CAD build for the part. Positions are in the model's coordinates, mm. Give positions to 0.01 mm unless a question says otherwise; leave off trailing zeros. Loops run counter-clockwise (first coordinate to the right, second up) from the corner with the lowest first, then second, coordinate; pieces in that order, holes last. Notation, with made-up numbers: M 80.25,-3 L 97.25,-3 A28 ccw 97.25,33 Z; hole C 58.5,64.5 d1. An arc over 180 degrees is marked long. Answer as CSV lines item,"result".
```python
from build123d import *

# Parameters (mm, degrees)
SKETCH1_R          = 5.4864
BASE_EXTRUDE_DEPTH = 0.635
SKETCH2_R          = 4.064
CUT_EXTRUDE1_DEPTH = 1.635
CUT_EXTRUDE4_DEPTH = 1.635
CIRPATTERN1_COUNT  = 14


with BuildPart() as part:
    # Sketch1 → Base-Extrude (new body)
    with BuildSketch(Plane.XY):
        Circle(SKETCH1_R)
    extrude(amount=BASE_EXTRUDE_DEPTH)

    # Sketch2 → Cut-Extrude1 (cut, through all)
    with BuildSketch(Plane.XY.offset(0.635)):
        Circle(SKETCH2_R)
    extrude(amount=-CUT_EXTRUDE1_DEPTH, mode=Mode.SUBTRACT)

    # Sketch3 → Cut-Extrude4 (cut, through all)
    with BuildSketch(Plane.XY.offset(0.635)):
        with BuildLine():
            Line((0.381, 4.04610121), (0.381, 4.3815))
            ThreePointArc((0.381, 4.3815), (0, 4.7625), (-0.381, 4.3815))
            Line((-0.381, 4.3815), (-0.381, 4.04610121))
            ThreePointArc((-0.381, 4.04610121), (0, 4.064), (0.381, 4.04610121))
        make_face()
    cut_extrude4 = extrude(amount=-CUT_EXTRUDE4_DEPTH, mode=Mode.SUBTRACT)

    # CirPattern1: Cut-Extrude4 ×14 about axis
    cirpattern1_axis = Axis((0, 0, 0), (0, 0, 1))
    for i in range(1, CIRPATTERN1_COUNT):
        add(cut_extrude4.rotate(cirpattern1_axis, i * 360 / CIRPATTERN1_COUNT), mode=Mode.SUBTRACT)


solid = part.part
```
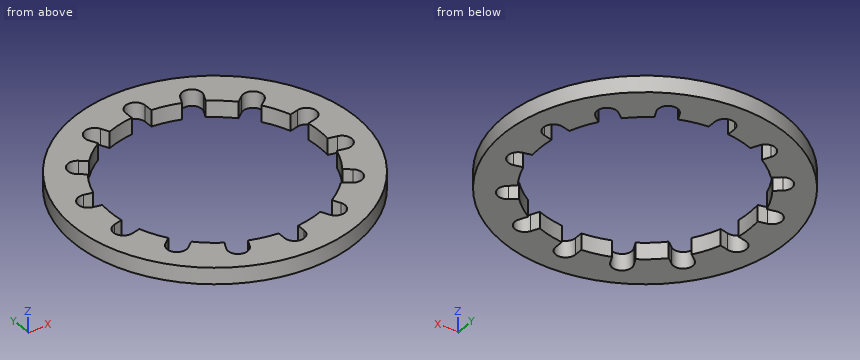
Q1. Wall check: line 1 (X direction, y = 4.25, z = 0.4); line 2 (X direction, y = 3.25, z = 0.2); line 3 (Y direction, x = -3.5, z = 0.45) (3 decimals). Give the ranges that are in metal, low to high. Write a range as [from, to].
Solution:
line 1,"x = [-3.47, -2.13], [-1.67, -0.38], [0.38, 1.67], [2.13, 3.47]"
line 2,"x = [-4.42, -2.44], [2.44, 4.42]"
line 3,"y = [-4.225, -3.105], [-2.304, -2.065], [2.065, 2.304], [3.105, 4.225]"
Q2. Cut at C-C (x = -4.5). Write the cut outline in (y, z) (3 decimals).
Solution:
outline,"M -3.139,0 L -1.28,0 L -1.28,0.635 L -3.139,0.635 Z; M -0.67,0 L 0.67,0 L 0.67,0.635 L -0.67,0.635 Z; M 1.28,0 L 3.139,0 L 3.139,0.635 L 1.28,0.635 Z"
Q3. Cut at B-B (y = 0). Write the cut outline in (x, z) (3 decimals).
Solution:
outline,"M -5.486,0 L -4.064,0 L -4.064,0.635 L -5.486,0.635 Z; M 4.064,0 L 5.486,0 L 5.486,0.635 L 4.064,0.635 Z"
Q4. Cut at A-A (x = 0). Write the cut outline in (y, z) (1 decimal).
Solution:
outline,"M -5.5,0 L -4.8,0 L -4.8,0.6 L -5.5,0.6 Z; M 4.8,0 L 5.5,0 L 5.5,0.6 L 4.8,0.6 Z"
